The drawing under review shows one solid part. Ordinate dimensions are in mm from its lowest x, y, z. A direction names the side the tool comes from. Give positions to 0.01 mm unless a question says otherwise; leave off trailing zeros. Loops run counter-clockwise (first coordinate to the right, second up) from the corner with the lowest first, then second, coordinate; pieces in that order, holes last. Notation, with made-up numbers: M 40.25,-1 L 94.25,-1 A8 cw 94.25,4 Z; hole C 49.25,-6 d3. An arc over 180 degrees is marked long. One line per item, written item: value. Start each with the question number.
Q1. We need section D-D on x = 20. Write out the cut boundary in (y, z).
Q2. We need section A-A on y = 11. Write out the cut boundary in (x, z).
Q3. For pin 1 (2 mm diameter, centred on x = 22.5, z = 14.5, fed in from +Y); pin 2 (5.5 mm diameter, centred on x = 11, y = 24.5, fed in from -Z); pin 3 (5 mm diameter, centred on y = 22.5, z = 27, fed in from +X), all flat-tipped, find the tip position at first contact; note any pin that passes through.
Q4. For the marked faces 1 and 2, list the 3-axis set-ups (+Z, -Z, +X, -X, +Y, -Y) from which the entire face can be reached by the end or side of a thin tool; tool diameter is ignored.
Q5. We need section C-C on z = 15. Write out the cut boundary in (x, y), plus the area to 3 significant figures.
Q6. We need section B-B on x = 11. Write out the cut boundary in (y, z), plus the area to 3 significant figures.
Q7. To check wall thickness, follow line 1 along Y through (x, z) = (10, 14); line 2 along Z through (x, y) = (4, 28.5); line 3 along X through (y, z) = (7, 7). State the ranges of each line that lie inside material, in increasing order. Write a range as from..to.
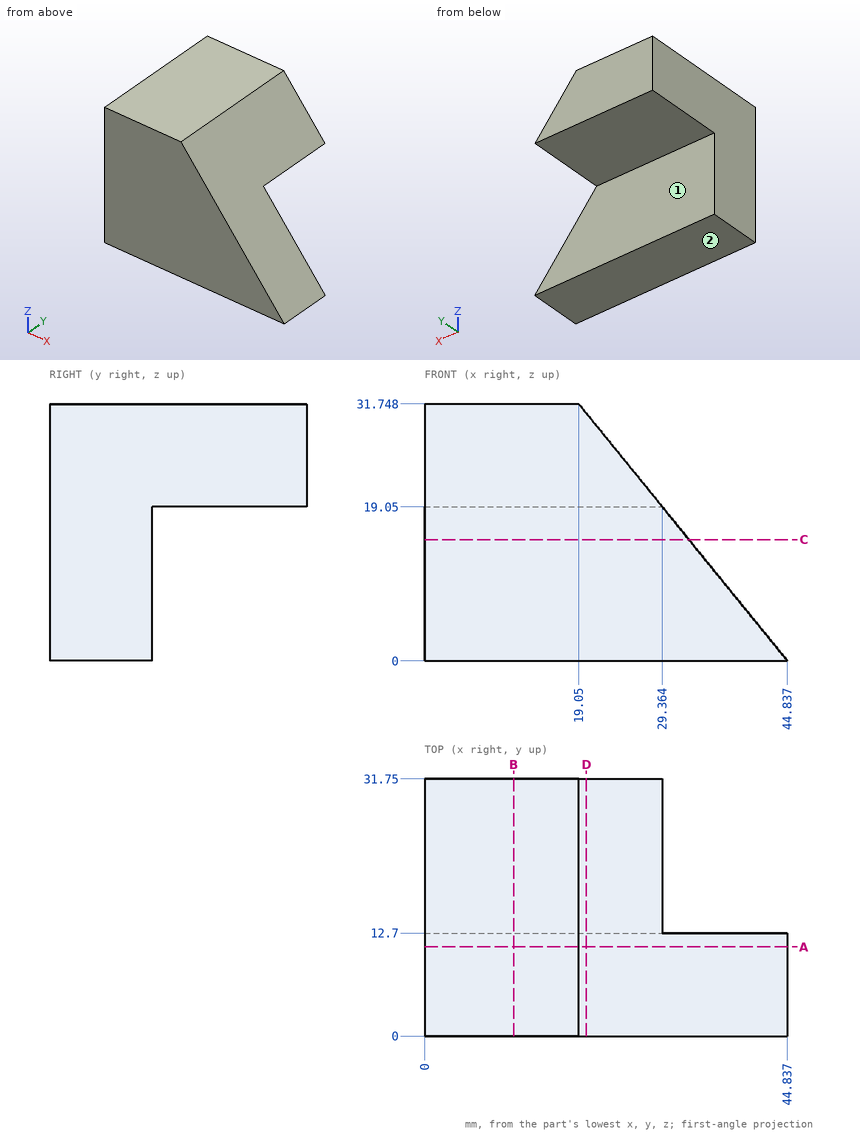
Solved:
1. outline: M 0,0 L 12.7,0 L 12.7,19.05 L 31.75,19.05 L 31.75,30.58 L 0,30.58 Z
2. outline: M 0,0 L 44.84,0 L 19.05,31.75 L 0,31.75 Z
3. pin 1: y = 12.7
3. pin 2: z = 19.05
3. pin 3: x = 24.94
4. face 1: -Z, +X, -X, +Y
4. face 2: -Z, +X, -X, +Y, -Y
5. outline: M 0,0 L 32.65,0 L 32.65,12.7 L 0,12.7 Z
5. area: 415 mm2
6. outline: M 0,0 L 12.7,0 L 12.7,19.05 L 31.75,19.05 L 31.75,31.75 L 0,31.75 Z
6. area: 645 mm2
7. line 1: 0..12.7
7. line 2: 19.05..31.75
7. line 3: 0..39.15
